Input: part model. Units: mm. Frame: model coordinates. A direction names the side the tool comes from. Coordinates: 2 decimals unless noted, no trailing zeros. Order: outer loops, then holes, each group sorted by start corner. A loop starts at its lowest first (then second) coordinate and runs counter-clockwise, first axis right, second up. Notation, with made-up numbers: M 81.5,-37 L 88.5,-37 A30 ccw 88.5,-4 Z; hole C 67.25,11 d10. An arc over 180 degrees is marked long. Answer in a Markdown table with one row per item.
from build123d import *

# Parameters (mm, degrees)
F0_W      = 35
F0_H      = 75
F1_DEPTH  = 2
F2_R      = 5.5
F3_DEPTH  = 75
F4_W      = 35
F4_H      = 75
F5_DEPTH  = 2
F7_R      = 3.5
F8_DEPTH  = 6.501
F9_R      = 3.5
F10_DEPTH = 6.501


with BuildPart() as f1:
    # F0 (on Front) → F1 (new body)
    with BuildSketch(Plane.XZ):
        Rectangle(F0_W, F0_H)
    extrude(amount=F1_DEPTH)


with BuildPart() as f3:
    # F2 (on face) → F3 (new body)
    with BuildSketch(Plane.XY.offset(37.5)):
        with Locations((-22.5, -1)):
            Circle(F2_R)
    extrude(amount=-F3_DEPTH)


with BuildPart() as f5:
    # F4 (on face) → F5 (new body)
    with BuildSketch(Plane.XZ.offset(2)):
        with Locations((-45, 0)):
            Rectangle(F4_W, F4_H)
    extrude(amount=-F5_DEPTH)


with BuildPart() as f1_1:
    add(f1.part)

    # F6: union F3, F5
    add(f3.part)
    add(f5.part)

    # F7 (on face) → F8 (cut, through all)
    with BuildSketch(Plane.XZ.offset(2)):
        with Locations((1.908327, -29.5)):
            Circle(F7_R)
        with Locations((1.908327, 29.5)):
            Circle(F7_R)
        with Locations((7.5, 0)):
            Circle(F7_R)
    extrude(amount=-F8_DEPTH, mode=Mode.SUBTRACT)

    # F9 (on face) → F10 (cut, through all)
    with BuildSketch(Plane.XZ.offset(2)):
        with Locations((-46.908327, -29.5)):
            Circle(F9_R)
        with Locations((-46.908327, 29.5)):
            Circle(F9_R)
        with Locations((-52.5, 0)):
            Circle(F9_R)
    extrude(amount=-F10_DEPTH, mode=Mode.SUBTRACT)


solid = f1_1.part
1) Mould query, pull axis Z, two halves, no side actions, for faces 1 (the face through (4, -1, 0)), 2 (the face through (1.45, -1.01, 32.97)), 3 (the face through (-23, -1, -37.5)), 4 (the face through (-22.6, -6.5, 0.5)). Classes: +Z half, -Z half, draft (parallel to the pull), parting line (faces both ways), or undercut.
Resolved:
| item | result |
|---|---|
| face 1 | undercut |
| face 2 | undercut |
| face 3 | -Z half |
| face 4 | draft |
2) Cut plane A-A, the plane z = -29.5. Output: boundary loops of the cut face in (x, y).
Resolved:
| item | result |
|---|---|
| outline | M -62.5,-2 L -50.41,-2 L -50.41,0 L -62.5,0 Z; M -43.41,-2 L -27.91,-2 A5.5 ccw -17.09,-2 L -1.59,-2 L -1.59,0 L -17.09,0 A5.5 ccw -27.91,0 L -43.41,0 Z; M 5.41,-2 L 17.5,-2 L 17.5,0 L 5.41,0 Z |
3) Cut plane D-D, the plane z = 5. Output: boundary loops of the cut face in (x, y).
Resolved:
| item | result |
|---|---|
| outline | M -62.5,-2 L -27.91,-2 A5.5 ccw -17.09,-2 L 17.5,-2 L 17.5,0 L -17.09,0 A5.5 ccw -27.91,0 L -62.5,0 Z |
4) Material intervals for probe 1 along Z at (x, y) = (7.5, -0.55); probe 2 along Y at (x, z) = (-37, 8); probe 3 along X at (y, z) = (-4, 8), sorted ascending.
Resolved:
| item | result |
|---|---|
| probe 1 | z = -37.5 to -3.5, 3.5 to 37.5 |
| probe 2 | y = -2 to 0 |
| probe 3 | x = -27.11 to -17.89 |
5) Contact query for flat-ended pins moving along their axis: pin 1 (6 mm diameter, centred on y = 1, z = -13, fed in from +X); pin 2 (8 mm diameter, centred on x = 7.5, z = 0, fed in from +Y); pin 3 (4 mm diameter, centred on x = 1.91, z = -29.5, fed in from -Y); pin 4 (17.5 mm diameter, centred on x = -1, z = 2, fed in from -Y). Output: stop coordinate, or through.
Resolved:
| item | result |
|---|---|
| pin 1 | stops at x = 17.5 |
| pin 2 | stops at y = 0 |
| pin 3 | passes through |
| pin 4 | stops at y = -2 |
6) Cut plane C-C, the plane x = 1. Output: boundary loops of the cut face in (y, z), and give its area (3 significant figures).
Resolved:
| item | result |
|---|---|
| outline | M -2,-37.5 L 0,-37.5 L 0,-32.88 L -2,-32.88 Z; M -2,-26.12 L 0,-26.12 L 0,26.12 L -2,26.12 Z; M -2,32.88 L 0,32.88 L 0,37.5 L -2,37.5 Z |
| area | 123 mm2 |
7) Reachability of faces 5 (the face through (0, -2, 1)), 6 (the face through (-45, -2, 1)), 7 (the face through (-45, 0, 1)), 8 (the face through (0, 0, 1)) from +Z, -Z, +X, -X, +Y, -Y: full face, straight path, thin tool, end or side. Return the list, or none.
Resolved:
| item | result |
|---|---|
| face 5 | +Z, -Z, +X, -Y |
| face 6 | +Z, -Z, -X, -Y |
| face 7 | +Z, -Z, -X, +Y |
| face 8 | +Z, -Z, +X, +Y |
8) Cut plane B-B, the plane x = -52.5. Output: boundary loops of the cut face in (y, z).
Resolved:
| item | result |
|---|---|
| outline | M -2,-37.5 L 0,-37.5 L 0,-3.5 L -2,-3.5 Z; M -2,3.5 L 0,3.5 L 0,37.5 L -2,37.5 Z |
